from build123d import *

# Parameters (mm, degrees)
F0_R     = 123.825
F0_R_2   = 120.65
F1_DEPTH = 254
F2_R     = 123.825
F3_DEPTH = 3.175
F4_R     = 12.7


with BuildPart() as f1:
    # F0 (on Top) → F1 (new body)
    with BuildSketch(Plane.XY):
        Circle(F0_R)
        Circle(F0_R_2, mode=Mode.SUBTRACT)
    extrude(amount=-F1_DEPTH)

    # F2 (on face) → F3 (join)
    with BuildSketch(Plane(origin=(0, 0, -254), x_dir=(1, 0, 0), z_dir=(0, 0, -1))):
        Circle(F2_R)
    extrude(amount=-F3_DEPTH)

    # F4
    f4_edges = [f1.edges().sort_by_distance(p)[0] for p in [
        (-123.825, 0, -254),
        (-120.65, 0, -250.825),
    ]]
    fillet(f4_edges, radius=F4_R)


solid = f1.part
Work out the finished part from the listing and answer in its coordinate system (mm). A direction names the side the tool comes from. Round coordinates to 2 decimals unless told otherwise and drop trailing zeros. Order: outer loops, then holes, each group sorted by start corner. A loop starts at its lowest first (then second) coordinate and runs counter-clockwise, first axis right, second up. Notation, with made-up numbers: M -21.75,38.25 L 8.25,38.25 A16 cw 8.25,53.25 Z; hole C 63.5,47 d2. An arc over 180 degrees is marked long. Put each result on its own line as item: value. Start each with the question number.
Q1. A tool of negligible diameter and unlimited length cuts with its end or side. For faces 4 (the cylindrical face through (-120.533, 5.305, -117.396)), 5 (the flat face through (-2, 2, -254)), from which of +Z, -Z, +X, -X, +Y, -Y can it reach the whole face along a straight path? Write none if from no direction.
Q2. Straight lines are drawn through the part: L1, parallel to Y at x = 0, z = -111 (3 decimals); L2, parallel to Z at x = 12, y = 50.5 (3 decimals); L3, parallel to Y at x = 23, z = -105. For each, find the intervals that lie inside material, in ascending order. Write a range as [from, to].
Q3. Section A-A, the plane x = 0 is taken. Write down the section's boundary in (y, z) (3 decimals).
Q4. Flat-ended cylindrical pins translate along their axes: pin 1 (4 mm diameter, centred on y = 8.5, z = -169.5, fed in from +X); pin 2 (3 mm diameter, centred on x = 55, z = -167.5, fed in from -Y); pin 3 (4 mm diameter, centred on y = 79, z = -106, fed in from +X). Find the tip coordinate at first contact, or state that the pin passes through.
Q5. For a pull along X with two mould halves and no side action, classify faces 1 (the cylindrical face through (-26.84, -120.88, -118.96)), 2 (the flat face through (27, -119, 0)), 3 (the flat face through (-2, -2, -250.825)) as pulls with the +X half, pulls with the -X half, needs draft (parallel to the pull), parting line crosses it, or undercut.
Q6. Section B-B, the plane z = -226 is taken. Write down the section's boundary in (x, y) (3 decimals).
Findings below:
1. face 4: +Z
1. face 5: -Z, +X, -X, +Y, -Y
2. L1: y = [-123.825, -120.65], [120.65, 123.825]
2. L2: z = [-254, -250.825]
2. L3: y = [-121.67, -118.44], [118.44, 121.67]
3. outline: M -123.825,-241.3 A12.7 ccw -111.125,-254 L 111.125,-254 A12.7 ccw 123.825,-241.3 L 123.825,0 L 120.65,0 L 120.65,-238.125 A12.7 cw 107.95,-250.825 L -107.95,-250.825 A12.7 cw -120.65,-238.125 L -120.65,0 L -123.825,0 Z
4. pin 1: stops at x = 123.65
4. pin 2: stops at y = -111.67
4. pin 3: stops at x = 96.97
5. face 1: parting line crosses it
5. face 2: needs draft
5. face 3: undercut
6. outline: C 0,0 d247.65; hole C 0,0 d241.3
